Work out the finished part from the listing and answer in its coordinate system (mm). Coordinates: 2 decimals unless noted, no trailing zeros. Order: outer loops, then holes, each group sorted by start corner. A loop starts at its lowest first (then second) coordinate and runs counter-clockwise, first axis right, second up.
1. Flat-ended cylindrical pins translate along their axes: pin 1 Ø1.5 at (x, z) = (-5, 27) entering from -Y; pin 2 Ø10 at (x, z) = (6.5, 12) entering from +Y (3 decimals); pin 3 Ø3 at (x, z) = (14, 15) entering from +Y (3 decimals); pin 4 Ø3.5 at (x, y) = (15, 0) entering from +Z. Find the tip coordinate at first contact, or state that the pin passes through.
2. Find the intervals of material crossed by probe 1 along X at (y, z) = (-1, 33); probe 2 along Y at (x, z) = (-15, 18), in increasing order.
3. The part is cut by section C-C, the plane x = 15. Give the vertices of the cut face in (y, z), then the cut area to 3 significant figures.
4. Determine the mould class of faces 1 (the flat face through (-10, 10, 22)), 2 (the flat face through (10, -10, 22)), 3 (the cylindrical face through (-12, 0, 22)), 4 (the flat face through (7.92, 0.18, 42.23)) for opening direction Y: +Y half, -Y half, draft (parallel to the pull), parting line (faces both ways), or undercut.
5. The part is cut by section D-D, the plane y = -6.25. Give the vertices of the cut face in (x, z), then the cut area to 3 significant figures.
6. The part is cut by section B-B, the plane z = 28. Give the vertices of the cut face in (x, y), then the cut area to 3 significant figures.
7. The part is cut by section A-A, the plane y = 0. Give the vertices of the cut face in (x, z), then the cut area to 3 significant figures.
```python
from build123d import *

# Parameters (mm, degrees)
SKETCH1_W           = 40
SKETCH1_H           = 25
BOSS_EXTRUDE1_DEPTH = 45
CUT_EXTRUDE1_DEPTH  = 45
CUT_EXTRUDE2_DEPTH  = 45
SKETCH4_R           = 3
CUT_EXTRUDE3_DEPTH  = 51.806003582


with BuildPart() as part:
    # Sketch1 → Boss-Extrude1 (new body)
    with BuildSketch(Plane.XY):
        Rectangle(SKETCH1_W, SKETCH1_H)
    extrude(amount=BOSS_EXTRUDE1_DEPTH)

    # Sketch2 → Cut-Extrude1 (cut)
    with BuildSketch(Plane(origin=(0, 12.5, 0), x_dir=(1, 0, 0), z_dir=(0, 1, 0))):
        Polygon((0, -45), (-20, -38), (-20, -45), align=None)
        Polygon((20, -45), (20, -38), (0, -45), align=None)
        Polygon((20, 0), (0, 0), (20, -7), align=None)
        Polygon((0, 0), (-20, -7), (-20, 0), align=None)
    extrude(amount=-CUT_EXTRUDE1_DEPTH, mode=Mode.SUBTRACT)

    # Sketch3 → Cut-Extrude2 (cut)
    with BuildSketch(Plane.XY):
        Polygon((-20, 12.5), (0, 12.5), (-20, 7.5), align=None)
        Polygon((20, 12.5), (20, 7.5), (0, 12.5), align=None)
        Polygon((20, -12.5), (0, -12.5), (20, -7.5), align=None)
        Polygon((-20, -12.5), (-20, -7.5), (0, -12.5), align=None)
    extrude(amount=CUT_EXTRUDE2_DEPTH, mode=Mode.SUBTRACT)

    # Sketch4 → Cut-Extrude3 (cut, through all)
    with BuildSketch(Plane.XY):
        with Locations(Location((-15, 0, 0), (0, 0, 180))):
            Circle(SKETCH4_R)
        with Locations(Location((15, 0, 0), (0, 0, 180))):
            Circle(SKETCH4_R)
    extrude(amount=CUT_EXTRUDE3_DEPTH, mode=Mode.SUBTRACT)


solid = part.part
```
Geometry says:
1. pin 1: stops at y = -11.44
1. pin 2: stops at y = 12.125
1. pin 3: stops at y = 9.375
1. pin 4: passes through
2. probe 1: x = -20 to -17.83, -12.17 to 12.17, 17.83 to 20
2. probe 2: y = -8.75 to -3, 3 to 8.75
3. outline: (-8.75, 5.25) - (-3, 5.25) - (-3, 39.75) - (-8.75, 39.75) - close; (3, 5.25) - (8.75, 5.25) - (8.75, 39.75) - (3, 39.75) - close
3. area: 397 mm2
4. face 1: +Y half
4. face 2: -Y half
4. face 3: undercut
4. face 4: draft
5. outline: (-20, 7) - (0, 0) - (20, 7) - (20, 38) - (0, 45) - (-20, 38) - close
5. area: 1,520 mm2
6. outline: (-20, -7.5) - (0, -12.5) - (20, -7.5) - (20, 7.5) - (0, 12.5) - (-20, 7.5) - close; hole circle Ø6 at (-15, 0); hole circle Ø6 at (15, 0)
6. area: 743 mm2
7. outline: (-20, 7) - (-18, 6.3) - (-18, 38.7) - (-20, 38) - close; (-12, 4.2) - (0, 0) - (12, 4.2) - (12, 40.8) - (0, 45) - (-12, 40.8) - close; (18, 6.3) - (20, 7) - (20, 38) - (18, 38.7) - close
7. area: 1,110 mm2
